Build history of the part. All positions in model axes, mm. Round coordinates to 2 decimals unless told otherwise and drop trailing zeros. Write each loop counter-clockwise with the first axis right and the second up, starting at its lowest first coordinate (ties: lowest second). Pieces come first, ordered by that corner, then holes. Notation, with made-up numbers: (66, 1) - (106, 1) arc R17 cw to (106, 12) - close; hole circle Ø4 at (46.5, 85.5). An arc over 180 degrees is marked (long way). Answer as a JSON object with one key per item and string values. Group by question number.
Item 1: Probe line 1 (Y direction, x = 0.2, z = 0); line 2 (X direction, y = 41, z = 3); line 3 (Z direction, x = 6.5, y = 9.5). List the from-to ranges inside material, lowest first. Write a range as from..to.
Item 2: Flat gauge pins, fed straight in: pin 1 (2 mm diameter, centred on x = 42, z = 3, fed in from +Y); pin 2 (6 mm diameter, centred on y = -21.5, z = -0.5, fed in from +X); pin 3 (5 mm diameter, centred on y = 18, z = -2, fed in from +X); pin 4 (0.8 mm diameter, centred on x = 0.5, z = -1.5, fed in from +Y). Where does each tip first touch, or does it go through?
Item 3: Two-plate mould, pull along X, no slides. Class faces 1 (the cylindrical face through (39.959, 77.932, 0.014)), 2 (the flat face through (0, 1, 0)), 3 (the flat face through (15, 33, -1)): +X half, -X half, draft (parallel to the pull), parting line (faces both ways), or undercut.
Item 4: Slice it at A-A, the plane z = -2.5. List the corners of the cut face in (x, y), then the cut area to 3 significant figures.
from build123d import *

# Parameters (mm, degrees)
SKETCH_1_W           = 10
SKETCH_1_H           = 100
EXTRUDE_1_DEPTH      = 1
SKETCH_2_W           = 2
SKETCH_2_H           = 30
SKETCH_2_H_2         = 10
SKETCH_2_H_3         = 80
EXTRUDE_3_DEPTH      = 50
SKETCH_3_R           = 8
CUT_EXTRUDE_11_DEPTH = 50
SKETCH_4_R           = 1
CUT_EXTRUDE_12_DEPTH = 1
SKETCH_5_R           = 1
CUT_EXTRUDE_13_DEPTH = 1


with BuildPart() as part:
    # 草图1 → 凸台-拉伸1 (new body)
    with BuildSketch(Plane(origin=(0, 0, 0), x_dir=(0, 0, -1), z_dir=(1, 0, 0))):
        Rectangle(SKETCH_1_W, SKETCH_1_H)
    extrude(amount=EXTRUDE_1_DEPTH)

    # 草图2 → 凸台-拉伸3 (add)
    with BuildSketch(Plane(origin=(1, 0, 0), x_dir=(0, 0, -1), z_dir=(1, 0, 0))):
        with Locations((0, 65)):
            Rectangle(SKETCH_2_W, SKETCH_2_H)
        with Locations((0, 45)):
            Rectangle(SKETCH_2_W, SKETCH_2_H_2)
        Rectangle(SKETCH_2_W, SKETCH_2_H_3)
    extrude(amount=EXTRUDE_3_DEPTH)

    # 草图3 → 切除-拉伸11 (cut)
    with BuildSketch(Plane.XY.offset(1)):
        with BuildLine():
            Line((1, 80), (1, 40))
            add(Edge.make_bspline(
                [(1, 40), (9.468575597, 40.414680021), (30.950220462, 58.157084532), (31.024773588, 69.296538532)],
                knots=[0, 0, 0, 0, 0.979118635, 0.979118635, 0.979118635, 0.979118635], degree=3))
            ThreePointArc((31.024773588, 69.296538532), (33.684447571, 76.817821695), (41, 80))
            Line((41, 80), (1, 80))
        make_face()
        with Locations((41, 70)):
            Circle(SKETCH_3_R)
        with BuildLine():
            add(Edge.make_bspline(
                [(1, -40), (4.194748365, 9.503139803), (28.570241109, 58.174536765), (42.100694242, 60.060760986)],
                knots=[0, 0, 0, 0, 1, 1, 1, 1], degree=3))
            Line((1, -40), (51, -40))
            Line((51, -40), (51, 70))
            ThreePointArc((51, 70), (48.450065182, 63.329428151), (42.100694242, 60.060760986))
        make_face()
        with BuildLine():
            Line((51, 80), (41, 80))
            ThreePointArc((41, 80), (48.071067812, 77.071067812), (51, 70))
            Line((51, 70), (51, 80))
        make_face()
    extrude(amount=-CUT_EXTRUDE_11_DEPTH, mode=Mode.SUBTRACT)

    # 草图4 → 切除-拉伸12 (cut)
    with BuildSketch(Plane.ZY):
        with Locations((0, 44.964354978)):
            Circle(SKETCH_4_R)
    extrude(amount=-CUT_EXTRUDE_12_DEPTH, mode=Mode.SUBTRACT)

    # 草图5 → 切除-拉伸13 (cut)
    with BuildSketch(Plane.ZY):
        with Locations((0, -45)):
            Circle(SKETCH_5_R)
    extrude(amount=-CUT_EXTRUDE_13_DEPTH, mode=Mode.SUBTRACT)


solid = part.part
Geometry says:
{
 "1": {"line 1": "y = -50..-46, -44..43.96, 45.96..50", "line 2": "x = 0..1", "line 3": "z = -1..1"},
 "2": {"pin 1": "passes through", "pin 2": "stops at x = 3.66", "pin 3": "stops at x = 14.54", "pin 4": "stops at y = 50"},
 "3": {"face 1": "undercut", "face 2": "-X half", "face 3": "draft"},
 "4": {"outline": "(0, -50) - (1, -50) - (1, 50) - (0, 50) - close", "area": "100 mm^2"}
}
